from build123d import *

# Parameters (mm, degrees)
BOSS_EXTRUDE1_DEPTH       = 18
F_1_0MM_DOWEL_HOLE3_D     = 9
SKETCH12_W                = 20
SKETCH12_H                = 20
CUT_EXTRUDE2_DEPTH        = 6
CUT_EXTRUDE3_DEPTH        = 12
CUT_EXTRUDE4_DEPTH        = 43
F_1_0MM_DOWEL_HOLE4_D     = 6
F_1_0MM_DOWEL_HOLE4_DEPTH = 6
F_1_0MM_DOWEL_HOLE4_TIP   = 1.802581857


with BuildPart() as part:
    # Sketch2 → Boss-Extrude1 (new body, symmetric)
    with BuildSketch(Plane.XY):
        with BuildLine():
            Line((18.761663039, 3), (22, 3))
            Line((22, 3), (22, 16))
            Line((22, 16), (50, 16))
            Line((50, 16), (50, -27))
            Line((50, -27), (79, -27))
            Line((79, -27), (82, -38))
            Line((82, -38), (-82, -38))
            Line((-82, -38), (-79, -27))
            Line((-79, -27), (-50, -27))
            Line((-50, -27), (-50, 16))
            Line((-50, 16), (-22, 16))
            Line((-22, 16), (-22, 3))
            Line((-22, 3), (-18.761663039, 3))
            ThreePointArc((-18.761663039, 3), (0, -19), (18.761663039, 3))
        make_face()
    extrude(amount=BOSS_EXTRUDE1_DEPTH, both=True)

    # Ø1.0mm Dowel Hole3 (through all)
    with Locations(Plane(origin=(0, 16, 0), x_dir=(1, 0, 0), z_dir=(0, 1, 0))):
        with Locations((-31, 0), (31, 0)):
            Hole(F_1_0MM_DOWEL_HOLE3_D / 2)

    # Sketch12 → Cut-Extrude2 (cut)
    with BuildSketch(Plane.XZ.offset(38)):
        with Locations((-31, 0)):
            Rectangle(SKETCH12_W, SKETCH12_H)
    cut_extrude2 = extrude(amount=-CUT_EXTRUDE2_DEPTH, mode=Mode.SUBTRACT)

    # Sketch13 → Cut-Extrude3 (cut, through all)
    with BuildSketch(Plane(origin=(0, -27, 0), x_dir=(1, 0, 0), z_dir=(0, 1, 0))):
        with BuildLine():
            Line((-67.5, 4.5), (-60.5, 4.5))
            ThreePointArc((-60.5, 4.5), (-56, 0), (-60.5, -4.5))
            Line((-60.5, -4.5), (-67.5, -4.5))
            ThreePointArc((-67.5, -4.5), (-72, 0), (-67.5, 4.5))
        make_face()
        with BuildLine():
            Line((60.5, 4.5), (67.5, 4.5))
            ThreePointArc((67.5, 4.5), (72, 0), (67.5, -4.5))
            Line((67.5, -4.5), (60.5, -4.5))
            ThreePointArc((60.5, -4.5), (56, 0), (60.5, 4.5))
        make_face()
    extrude(amount=-CUT_EXTRUDE3_DEPTH, mode=Mode.SUBTRACT)

    # Mirror1: Cut-Extrude2 across plane
    add(cut_extrude2.mirror(Plane(origin=(0, 0, 0), x_dir=(0, 0, 1), z_dir=(1, 0, 0))), mode=Mode.SUBTRACT)

    # Sketch17 → Cut-Extrude4 (cut)
    with BuildSketch(Plane(origin=(0, 16, 0), x_dir=(1, 0, 0), z_dir=(0, 1, 0))):
        with BuildLine():
            Line((-44.497190923, 18), (-50, 18))
            Line((-50, 18), (-50, -18))
            Line((-50, -18), (-44.497190923, -18))
            ThreePointArc((-44.497190923, -18), (-48, 0), (-44.497190923, 18))
        make_face()
    cut_extrude4 = extrude(amount=-CUT_EXTRUDE4_DEPTH, mode=Mode.SUBTRACT)

    # Mirror3: Cut-Extrude4 across plane
    add(cut_extrude4.mirror(Plane(origin=(0, 0, 0), x_dir=(0, 0, 1), z_dir=(1, 0, 0))), mode=Mode.SUBTRACT)

    # Ø1.0mm Dowel Hole4
    with Locations(Plane(origin=(0, -19, 0), x_dir=(1, 0, 0), z_dir=(0, 1, 0))):
        with Locations((0, 0)):
            Hole(F_1_0MM_DOWEL_HOLE4_D / 2, depth=F_1_0MM_DOWEL_HOLE4_DEPTH)
            with Locations((0, 0, -(F_1_0MM_DOWEL_HOLE4_DEPTH + F_1_0MM_DOWEL_HOLE4_TIP / 2))):  # 118° drill point
                Cone(0, F_1_0MM_DOWEL_HOLE4_D / 2, F_1_0MM_DOWEL_HOLE4_TIP, mode=Mode.SUBTRACT)


solid = part.part
Part model, mm, in its own coordinate system. A direction names the side the tool comes from. Coordinates: 2 decimals unless noted, no trailing zeros. Order: outer loops, then holes, each group sorted by start corner. A loop starts at its lowest first (then second) coordinate and runs counter-clockwise, first axis right, second up.
(1) Slice it at C-C, the plane y = -28.5. Write the cut outline in (x, z).
Check sheet entries:
outline: (-79.41, -18) - (79.41, -18) - (79.41, 18) - (-79.41, 18) - close; hole (-67.5, -4.5) - (-60.5, -4.5) arc R4.5 ccw to (-60.5, 4.5) - (-67.5, 4.5) arc R4.5 ccw to start; hole circle Ø9 at (-31, 0); hole circle Ø9 at (31, 0); hole (60.5, -4.5) - (67.5, -4.5) arc R4.5 ccw to (67.5, 4.5) - (60.5, 4.5) arc R4.5 ccw to start
(2) Tool access for faces 1 (the face through (-56, -32, 0)), 2 (the face through (-41, -35, 0)), 3 (the face through (22, 9, 0)): list every direction of +Z, -Z, +X, -X, +Y, -Y with a clear straight run to the whole face (end or side of a thin tool).
Check sheet entries:
face 1: +Y, -Y
face 2: -Y
face 3: +Z, -Z, +Y
(3) Probe L1, parallel to Z at x = -31, y = -2.5; L2, parallel to X at y = -8.5, z = -2.5; L3, parallel to X at y = -31, z = -3. List the from-to ranges inside material, lowest first.
Check sheet entries:
L1: z = -18 to -4.5, 4.5 to 18
L2: x = -47.93 to -34.74, -27.26 to -16.99, 16.99 to 27.26, 34.74 to 47.93
L3: x = -80.09 to -70.85, -57.15 to -34.35, -27.65 to 27.65, 34.35 to 57.15, 70.85 to 80.09
(4) Slice it at D-D, the plane z = 15. Write the cut outline in (x, y).
Check sheet entries:
outline: (-82, -38) - (82, -38) - (79, -27) - (45.6, -27) - (45.6, 16) - (22, 16) - (22, 3) - (18.76, 3) arc R19 cw (long way) to (-18.76, 3) - (-22, 3) - (-22, 16) - (-45.6, 16) - (-45.6, -27) - (-79, -27) - close
(5) Slice it at A-A, the plane y = 9. Write the cut outline in (x, z).
Check sheet entries:
outline: (-44.5, -18) - (-22, -18) - (-22, 18) - (-44.5, 18) arc R48 ccw to start; (22, -18) - (44.5, -18) arc R48 ccw to (44.5, 18) - (22, 18) - close; hole circle Ø9 at (-31, 0); hole circle Ø9 at (31, 0)
(6) Slice it at B-B, the plane x = -31. Write the cut outline in (y, z), and give its area (3 significant figures).
Check sheet entries:
outline: (-38, -18) - (16, -18) - (16, -4.5) - (-32, -4.5) - (-32, -10) - (-38, -10) - close; (-38, 10) - (-32, 10) - (-32, 4.5) - (16, 4.5) - (16, 18) - (-38, 18) - close
area: 1,390 mm2
(7) Pull direction Z, two halves, no side cores. Call faces 4 (the face through (1, -23, -18)), 5 (the face through (-72, -32, 0)), 6 (the face through (1, -38, 0)): pulls with the +Z half, pulls with the -Z half, needs draft (parallel to the pull), parting line crosses it, or undercut.
Check sheet entries:
face 4: pulls with the -Z half
face 5: undercut
face 6: needs draft
(8) Pin check, flat tips, straight feed: pin 1 Ø3 at (y, z) = (-35.5, -2.5) entering from -X; pin 2 Ø14.5 at (y, z) = (7, -8) entering from -X; pin 3 Ø6 at (y, z) = (-16.5, -14) entering from +X; pin 4 Ø5.5 at (x, z) = (-31, 0) entering from -Y. Stop position of each tip, or through.
Check sheet entries:
pin 1: stops at x = -81.73
pin 2: stops at x = -47.99
pin 3: stops at x = 46.72
pin 4: passes through
